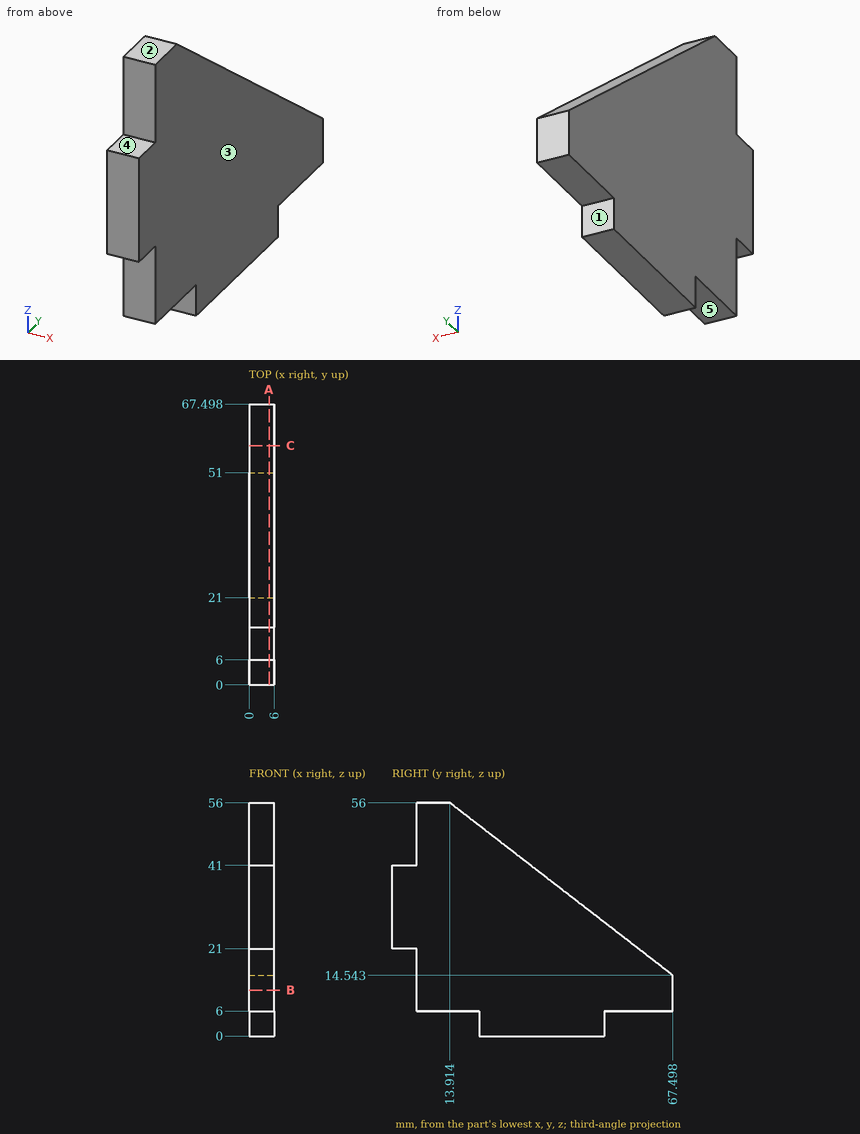
Verification items for this drawing (mm, ordinates from the low corner). A direction names the side the tool comes from. Give positions to 0.01 mm unless a question says otherwise; leave off trailing zeros. Loops run counter-clockwise (first coordinate to the right, second up) from the corner with the lowest first, then second, coordinate; pieces in that order, holes last. Notation, with made-up numbers: M 53,-39 L 57,-39 A25 ccw 57,-8 Z; hole C 47.25,82 d8. An arc over 180 degrees is marked long. Answer as a JSON object with one key per item and string values. Group by question number.
Item 1: Sectioned sample at B-B on z = 11. Record the boundary of the cut face in (x, y), plus the area to 3 significant figures.
Item 2: Material ranges on L1, parallel to Y at x = 3.4, z = 3.5; L2, parallel to Y at x = 1.1, z = 14; L3, parallel to Z at x = 1.3, y = 8, recorded low to high.
Item 3: Access from +Z, -Z, +X, -X, +Y, -Y to the whole of each face (thin tool, end or side, straight path). Record for the marked faces 1, 2, 3, 4 and 5.
Item 4: Gauge pin test, flat ends, axial feed: pin 1 (1.8 mm diameter, centred on x = 4, y = 57, fed in from -Z); pin 2 (1.5 mm diameter, centred on x = 3.5, y = 20.5, fed in from +Z) (1 decimal); pin 3 (3 mm diameter, centred on x = 2.5, z = 13.5, fed in from -Y). Record the tip position at first contact, or that the pin passes through.
Item 5: Sectioned sample at A-A on x = 4.8. Record the boundary of the cut face in (y, z) (1 decimal).
Item 6: Sectioned sample at C-C on y = 57.5. Record the boundary of the cut face in (x, z).
Findings below:
{
 "1": {"outline": "M 0,6 L 6,6 L 6,67.5 L 0,67.5 Z", "area": "369 mm2"},
 "2": {"L1": "21 to 51", "L2": "6 to 67.5", "L3": "6 to 56"},
 "3": {"face 1": "-Z, +X, -X, +Y", "face 2": "+Z, +X, -X, +Y, -Y", "face 3": "+Z, -Z, +X, +Y, -Y", "face 4": "+Z, +X, -X, -Y", "face 5": "-Z, +X, -X, -Y"},
 "4": {"pin 1": "z = 6", "pin 2": "z = 51.5", "pin 3": "y = 6"},
 "5": {"outline": "M 0,21 L 6,21 L 6,6 L 21,6 L 21,0 L 51,0 L 51,6 L 67.5,6 L 67.5,14.5 L 13.9,56 L 6,56 L 6,41 L 0,41 Z"},
 "6": {"outline": "M 0,6 L 6,6 L 6,22.28 L 0,22.28 Z"}
}
